The model under review builds one solid part; all positions refer to its coordinate system, in mm. Face numbers are marked on the shaded views. A direction names the side the tool comes from. Round coordinates to 2 decimals unless told otherwise and drop trailing zeros. Loops run counter-clockwise (first coordinate to the right, second up) from the corner with the lowest first, then second, coordinate; pieces in that order, holes last. Notation, with made-up numbers: (50.5, -17.5) -> (54.5, -17.5) arc R23 cw to (54.5, 17.5) -> close; hole circle Ø8 at (-35.5, 37). An arc over 180 degrees is marked (long way). Use a Markdown table: item, result. Add a question column.
1) Consider section C-C on z = 43. Give the boundary of the cut face in (x, y).
2) Consider section B-B on z = -376. Give the boundary of the cut face in (x, y), plus the area to 3 significant figures.
3) Wall thickness on probe 1 along Y at (x, z) = (172.5, 465.25); probe 2 along X at (y, z) = (35, 465.5); probe 3 along Y at (x, z) = (172.5, 468.25): over which ranges is each line inside the solid? List them lowest first.
4) Mouldability with a two-part tool opening along X and no side actions: class the marked faces 1, 2 and 3 as released by +X, released by -X, zero draft, split by the parting line, or undercut.
5) For the marked faces 4, 5, 6, 7 and 8, list the 3-axis set-ups (+Z, -Z, +X, -X, +Y, -Y) from which the entire face can be reached by the end or side of a thin tool; tool diameter is ignored.
6) Insertion check: pin 1 (3 mm diameter, centred on y = 134, z = 299.5, fed in from -X); pin 2 (5 mm diameter, centred on y = 16, z = -373, fed in from -X); pin 3 (8 mm diameter, centred on x = 153.5, y = 10, fed in from +Z). Each pin has a flat end and moves straight along its axis. Give the tip position at first contact, or say it passes through.
7) Consider section A-A on x = 503. Give the boundary of the cut face in (y, z).
from build123d import *

# Parameters (mm, degrees)
BOSS_EXTRUDE1_DEPTH               = 150
BOSS_EXTRUDE2_START               = 1.5
BOSS_EXTRUDE2_DEPTH               = 147
BOSS_EXTRUDE2_2_DEPTH             = 16
BOSS_EXTRUDE2_START_2             = 132.5
BOSS_EXTRUDE2_3_DEPTH             = 16
BOSS_EXTRUDE3_START               = -15
SKETCH3_W                         = 370
SKETCH3_H                         = 115
BOSS_EXTRUDE3_DEPTH               = 20
TAP_DRILL_FOR_M12_TAP1_AT_2_COUNT = 2
TAP_DRILL_FOR_M12_TAP1_AT_2_PITCH = 80
TAP_DRILL_FOR_M12_TAP1_AT_3_COUNT = 2
TAP_DRILL_FOR_M12_TAP1_AT_3_PITCH = 185
TAP_DRILL_FOR_M12_TAP1_AT_4_COUNT = 2
TAP_DRILL_FOR_M12_TAP1_AT_4_PITCH = 201.556443707
TAP_DRILL_FOR_M12_TAP1_AT_5_COUNT = 2
TAP_DRILL_FOR_M12_TAP1_AT_5_PITCH = 189.274932307
TAP_DRILL_FOR_M12_TAP1_AT_6_COUNT = 2
TAP_DRILL_FOR_M12_TAP1_AT_6_PITCH = 40


# Read off the part's stored shape, not the designer's step: Boss-Extrude2
with BuildPart() as part:
    # Sketch1 → Boss-Extrude1 (new body)
    with BuildSketch(Plane(origin=(0, 0, 0), x_dir=(1, 0, 0), z_dir=(0, 1, 0))):
        with BuildLine():
            Line((799.081072199, 213), (370.081072199, 213))
            ThreePointArc((370.081072199, 213), (-427, 0), (370.081072199, -213))
            Line((370.081072199, -213), (799.081072199, -213))
            Line((799.081072199, -213), (799.081072199, 213))
        make_face()
        with BuildLine():
            Line((355.330831761, 188), (774.081072199, 188))
            Line((774.081072199, 188), (774.081072199, -188))
            Line((774.081072199, -188), (355.330831761, -188))
            ThreePointArc((355.330831761, -188), (-402, 0), (355.330831761, 188))
        make_face(mode=Mode.SUBTRACT)
    extrude(amount=BOSS_EXTRUDE1_DEPTH)

    # Boss-Extrude2 outline → Boss-Extrude2 (add)
    with BuildSketch(Plane(origin=(0, 0, 0), x_dir=(1, 0, 0), z_dir=(0, 1, 0)).offset(BOSS_EXTRUDE2_START)):
        with BuildLine():
            Line((249, -467), (265, -467))
            Line((265, -467), (265, -334.819354279))
            ThreePointArc((265, -334.819354279), (257.070777199, -340.945179626), (249, -346.883265667))
            Line((249, -346.883265667), (249, -467))
        make_face()
        with BuildLine():
            Line((-105, -467), (-89, -467))
            Line((-89, -467), (-89, -417.621838509))
            ThreePointArc((-89, -417.621838509), (-97.017955844, -415.83231746), (-105, -413.888873975))
            Line((-105, -413.888873975), (-105, -467))
        make_face()
    boss_extrude2 = extrude(amount=BOSS_EXTRUDE2_DEPTH)

    # Boss-Extrude2 2 outline → Boss-Extrude2 2 (add)
    with BuildSketch(Plane(origin=(0, 0, 0), x_dir=(1, 0, 0), z_dir=(0, 1, 0)).offset(BOSS_EXTRUDE2_START)):
        with BuildLine():
            Line((-89, -467), (249, -467))
            Line((249, -467), (249, -346.883265667))
            ThreePointArc((249, -346.883265667), (87.46991724, -417.944988698), (-89, -417.621838509))
            Line((-89, -417.621838509), (-89, -467))
        make_face()
    boss_extrude2_2 = extrude(amount=BOSS_EXTRUDE2_2_DEPTH)

    # Boss-Extrude2 3 outline → Boss-Extrude2 3 (add)
    with BuildSketch(Plane(origin=(0, 0, 0), x_dir=(1, 0, 0), z_dir=(0, 1, 0)).offset(BOSS_EXTRUDE2_START_2)):
        with BuildLine():
            Line((-89, -467), (249, -467))
            Line((249, -467), (249, -346.883265667))
            ThreePointArc((249, -346.883265667), (87.46991724, -417.944988698), (-89, -417.621838509))
            Line((-89, -417.621838509), (-89, -467))
        make_face()
    boss_extrude2_3 = extrude(amount=BOSS_EXTRUDE2_3_DEPTH)

    # Sketch3 → Boss-Extrude3 (add)
    with BuildSketch(Plane.XY.offset(467).offset(BOSS_EXTRUDE3_START)):
        with Locations((80, 75)):
            Rectangle(SKETCH3_W, SKETCH3_H)
    boss_extrude3 = extrude(amount=BOSS_EXTRUDE3_DEPTH)

    # Sketch7 → Tap Drill for M12 Tap1 (revolve, cut)
    with BuildSketch(Plane(origin=(172.5, 115, 472), x_dir=(0, -1, 0), z_dir=(1, 0, 0))):
        Polygon((0, 0), (0, 16), (5.2, 12.875524781), (5.2, 0), align=None)
    tap_drill_for_m12_tap1 = revolve(axis=Axis((172.5, 115, 478.35), (0, 0, -1)), mode=Mode.SUBTRACT)

    # Tap Drill for M12 Tap1 at 2: Tap Drill for M12 Tap1 ×2
    with Locations(*[(0, -i * TAP_DRILL_FOR_M12_TAP1_AT_2_PITCH, 0) for i in range(1, TAP_DRILL_FOR_M12_TAP1_AT_2_COUNT)]):
        add(tap_drill_for_m12_tap1, mode=Mode.SUBTRACT)

    # Tap Drill for M12 Tap1 at 3: Tap Drill for M12 Tap1 ×2
    with Locations(*[(-i * TAP_DRILL_FOR_M12_TAP1_AT_3_PITCH, 0, 0) for i in range(1, TAP_DRILL_FOR_M12_TAP1_AT_3_COUNT)]):
        add(tap_drill_for_m12_tap1, mode=Mode.SUBTRACT)

    # Tap Drill for M12 Tap1 at 4: Tap Drill for M12 Tap1 ×2
    with Locations(*[Vector(-0.9178570359601427, -0.3969111506854671, 0) * (i * TAP_DRILL_FOR_M12_TAP1_AT_4_PITCH) for i in range(1, TAP_DRILL_FOR_M12_TAP1_AT_4_COUNT)]):
        add(tap_drill_for_m12_tap1, mode=Mode.SUBTRACT)

    # Tap Drill for M12 Tap1 at 5: Tap Drill for M12 Tap1 ×2
    with Locations(*[Vector(-0.9774141654398674, -0.21133279252753864, 0) * (i * TAP_DRILL_FOR_M12_TAP1_AT_5_PITCH) for i in range(1, TAP_DRILL_FOR_M12_TAP1_AT_5_COUNT)]):
        add(tap_drill_for_m12_tap1, mode=Mode.SUBTRACT)

    # Tap Drill for M12 Tap1 at 6: Tap Drill for M12 Tap1 ×2
    with Locations(*[(0, -i * TAP_DRILL_FOR_M12_TAP1_AT_6_PITCH, 0) for i in range(1, TAP_DRILL_FOR_M12_TAP1_AT_6_COUNT)]):
        add(tap_drill_for_m12_tap1, mode=Mode.SUBTRACT)

    # Mirror1: Boss-Extrude2, Boss-Extrude2 2, Boss-Extrude2 3, Boss-Extrude3, Tap Drill for M12 Tap1 across plane
    add(boss_extrude2.mirror(Plane.XY))
    add(boss_extrude2_2.mirror(Plane.XY))
    add(boss_extrude2_3.mirror(Plane.XY))
    add(boss_extrude3.mirror(Plane.XY))
    add(tap_drill_for_m12_tap1.mirror(Plane.XY), mode=Mode.SUBTRACT)

    # Mirror1 copy 1 sketch → Mirror1 copy 1 (revolve, cut)
    with BuildSketch(Plane(origin=(172.5, 35, -472), x_dir=(0, -1, 0), z_dir=(1, 0, 0))):
        Polygon((0, 0), (0, -16), (5.2, -12.875524781), (5.2, 0), align=None)
    revolve(axis=Axis((172.5, 35, -478.35), (0, 0, -1)), mode=Mode.SUBTRACT)

    # Mirror1 copy 2 sketch → Mirror1 copy 2 (revolve, cut)
    with BuildSketch(Plane(origin=(-12.5, 115, -472), x_dir=(0, -1, 0), z_dir=(1, 0, 0))):
        Polygon((0, 0), (0, -16), (5.2, -12.875524781), (5.2, 0), align=None)
    revolve(axis=Axis((-12.5, 115, -478.35), (0, 0, -1)), mode=Mode.SUBTRACT)

    # Mirror1 copy 3 sketch → Mirror1 copy 3 (revolve, cut)
    with BuildSketch(Plane(origin=(-12.5, 35, -472), x_dir=(0, -1, 0), z_dir=(1, 0, 0))):
        Polygon((0, 0), (0, -16), (5.2, -12.875524781), (5.2, 0), align=None)
    revolve(axis=Axis((-12.5, 35, -478.35), (0, 0, -1)), mode=Mode.SUBTRACT)

    # Mirror1 copy 4 sketch → Mirror1 copy 4 (revolve, cut)
    with BuildSketch(Plane(origin=(-12.5, 75, -472), x_dir=(0, -1, 0), z_dir=(1, 0, 0))):
        Polygon((0, 0), (0, -16), (5.2, -12.875524781), (5.2, 0), align=None)
    revolve(axis=Axis((-12.5, 75, -478.35), (0, 0, -1)), mode=Mode.SUBTRACT)

    # Mirror1 copy 5 sketch → Mirror1 copy 5 (revolve, cut)
    with BuildSketch(Plane(origin=(172.5, 75, -472), x_dir=(0, -1, 0), z_dir=(1, 0, 0))):
        Polygon((0, 0), (0, -16), (5.2, -12.875524781), (5.2, 0), align=None)
    revolve(axis=Axis((172.5, 75, -478.35), (0, 0, -1)), mode=Mode.SUBTRACT)


solid = part.part
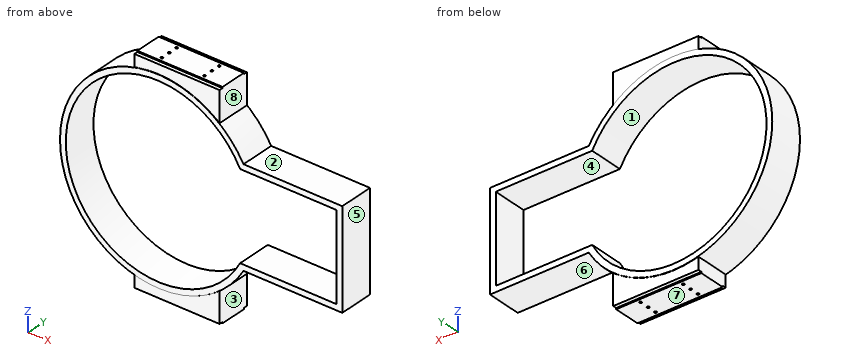
Result set:
| question | item | result |
|---|---|---|
| 1 | outline | (-424.83, 0) -> (-399.69, 0) -> (-399.69, 150) -> (-424.83, 150) -> close; (774.08, 0) -> (799.08, 0) -> (799.08, 150) -> (774.08, 150) -> close |
| 2 | outline | (-202.37, 0) -> (-142.23, 0) -> (-142.23, 150) -> (-202.37, 150) -> close; (142.23, 0) -> (202.37, 0) -> (202.37, 1.5) -> (265, 1.5) -> (265, 148.5) -> (202.37, 148.5) -> (202.37, 150) -> (142.23, 150) -> close; hole (202.37, 17.5) -> (249, 17.5) -> (249, 132.5) -> (202.37, 132.5) -> close |
| 2 | area | 21,900 mm2 |
| 3 | probe 1 | 1.5 to 29.8, 40.2 to 69.8, 80.2 to 109.8, 120.2 to 148.5 |
| 3 | probe 2 | -105 to -17.7, -7.3 to 167.3, 177.7 to 265 |
| 3 | probe 3 | 17.5 to 29.8, 40.2 to 69.8, 80.2 to 109.8, 120.2 to 132.5 |
| 4 | face 1 | undercut |
| 4 | face 2 | zero draft |
| 4 | face 3 | released by +X |
| 5 | face 4 | +Y, -Y |
| 5 | face 5 | +Z, -Z, +X, +Y, -Y |
| 5 | face 6 | -Z, +X, +Y, -Y |
| 5 | face 7 | -Z, +X, -X, +Y, -Y |
| 5 | face 8 | +Z, +X, +Y, -Y |
| 6 | pin 1 | x = -305.82 |
| 6 | pin 2 | x = -212.27 |
| 6 | pin 3 | z = 467 |
| 7 | outline | (0, -213) -> (150, -213) -> (150, -188) -> (0, -188) -> close; (0, 188) -> (150, 188) -> (150, 213) -> (0, 213) -> close |
